```python
from build123d import *

# Parameters (mm, degrees)
SKETCH1_R  = 1.5
BODY_DEPTH = 2.5


with BuildPart() as part:
    # Sketch1 → Body (new body)
    with BuildSketch(Plane.XY):
        with BuildLine():
            Line((10.7429859, -40.093369202), (12.099790359, -45.157032379))
            ThreePointArc((12.099790359, -45.157032379), (0, 46.75), (-12.099790359, -45.157032379))
            Line((-12.099790359, -45.157032379), (-10.7429859, -40.093369202))
            ThreePointArc((-10.7429859, -40.093369202), (-12.9932333, -35.397934549), (-17.977352649, -36.904345602))
            ThreePointArc((-17.977352649, -36.904345602), (-19.18898515, -37.770564542), (-20.663329885, -37.559149851))
            ThreePointArc((-20.663329885, -37.559149851), (0, 39.5), (20.663329885, -37.559149851))
            ThreePointArc((20.663329885, -37.559149851), (19.18898515, -37.770564542), (17.977352649, -36.904345602))
            ThreePointArc((17.977352649, -36.904345602), (12.9932333, -35.397934549), (10.7429859, -40.093369202))
        make_face()
        with Locations(Location((14.606689205, -39.058093022, 0), (0, 0, 180))):
            Circle(SKETCH1_R, mode=Mode.SUBTRACT)
        with Locations((-14.606689205, -39.058093022)):
            Circle(SKETCH1_R, mode=Mode.SUBTRACT)
    extrude(amount=-BODY_DEPTH)


solid = part.part
```
The listing builds one solid part. Answer for the finished solid, in the listing's coordinates (mm). A direction names the side the tool comes from. Round coordinates to 2 decimals unless told otherwise and drop trailing zeros. Write each loop counter-clockwise with the first axis right and the second up, starting at its lowest first coordinate (ties: lowest second). Pieces come first, ordered by that corner, then holes. Notation, with made-up numbers: (82, -1.5) -> (107, -1.5) arc R20 ccw to (107, 33.5) -> close; hole circle Ø4 at (64, 57). An arc over 180 degrees is marked (long way). Answer as a JSON object with one key per item and string values. Group by question number.
Q1. Section C-C (x = 39.5) is taken. Write down the section's boundary in (y, z).
Q2. Which of the six approach directions +Z, -Z, +X, -X, +Y, -Y give full straight-line access (tool end or side, diameter ignored) to faces 1 (the face through (-10.6, 38.5, -2.5)), 2 (the face through (11.41, -42.59, -1.23)), 3 (the face through (19.21, -37.776, -1.232))?
Q3. Straight lines are drawn through the part: line 1 along Y through (x, z) = (-19.5, -0.25); line 2 along X through (y, z) = (-24, -2.05); line 3 along X through (y, z) = (27, -0.9). For each, find the intervals that lie inside material, in ascending order.
Q4. Section A-A (y = 1.5) is taken. Write down the section's boundary in (x, z).
Q5. Section B-B (z = -1.75) is taken. Write down the section's boundary in (x, y).
Q6. Section D-D (x = 0) is taken. Write down the section's boundary in (y, z), plus the area to 3 significant figures.
Check values:
{
 "1": {"outline": "(-25.01, -2.5) -> (-13.86, -2.5) -> (-13.86, 0) -> (-25.01, 0) -> close; (10.26, -2.5) -> (25.01, -2.5) -> (25.01, 0) -> (10.26, 0) -> close"},
 "2": {"face 1": "-Z, +X, -X, +Y, -Y", "face 2": "+Z, -Z, -Y", "face 3": "+Z, -Z"},
 "3": {"line 1": "-42.49 to -37.82, 34.61 to 42.49", "line 2": "-40.12 to -34.83, 34.83 to 40.12", "line 3": "-38.16 to -29.6, 29.6 to 38.16"},
 "4": {"outline": "(-46.73, -2.5) -> (-41.17, -2.5) -> (-41.17, 0) -> (-46.73, 0) -> close; (41.17, -2.5) -> (46.73, -2.5) -> (46.73, 0) -> (41.17, 0) -> close"},
 "5": {"outline": "(-20.66, -37.56) arc R41.3 cw (long way) to (20.66, -37.56) arc R2 cw to (17.98, -36.9) arc R4 ccw to (10.74, -40.09) -> (12.1, -45.16) arc R46.75 ccw (long way) to (-12.1, -45.16) -> (-10.74, -40.09) arc R4 ccw to (-17.98, -36.9) arc R2 cw to start; hole circle Ø3 at (-14.61, -39.06); hole circle Ø3 at (14.61, -39.06)"},
 "6": {"outline": "(39.5, -2.5) -> (46.75, -2.5) -> (46.75, 0) -> (39.5, 0) -> close", "area": "18.1 mm^2"}
}
